from build123d import *

# Parameters (mm, degrees)
ESQUISSE1_R             = 0.9
ESQUISSE1_R_2           = 4
BOSS_EXTRU_1_DEPTH      = 6
ESQUISSE2_R             = 1.2
ENL_V_MAT_EXTRU_1_DEPTH = 10


with BuildPart() as part:
    # Esquisse1 → Boss.-Extru.1 (new body)
    with BuildSketch(Plane.XY):
        with BuildLine():
            Line((24.916434397, -77.573457495), (24.916434397, 1.426542505))
            Line((24.916434397, 1.426542505), (50.916434397, 1.426542505))
            Line((50.916434397, 1.426542505), (50.916434397, -77.573457495))
            ThreePointArc((50.916434397, -77.573457495), (49.159075085, -81.816098182), (44.916434397, -83.573457495))
            Line((44.916434397, -83.573457495), (30.916434397, -83.573457495))
            ThreePointArc((30.916434397, -83.573457495), (26.67379371, -81.816098182), (24.916434397, -77.573457495))
        make_face()
        with Locations((29.916434397, -68.573457495)):
            Circle(ESQUISSE1_R, mode=Mode.SUBTRACT)
        with Locations((37.916434397, -60.573457495)):
            Circle(ESQUISSE1_R, mode=Mode.SUBTRACT)
        with Locations((45.916434397, -68.573457495)):
            Circle(ESQUISSE1_R, mode=Mode.SUBTRACT)
        with Locations((37.916434397, -76.573457495)):
            Circle(ESQUISSE1_R, mode=Mode.SUBTRACT)
        with Locations((37.916434397, -68.573457495)):
            Circle(ESQUISSE1_R_2, mode=Mode.SUBTRACT)
    extrude(amount=BOSS_EXTRU_1_DEPTH)

    # Esquisse2 → Enlèv. mat.-Extru.1 (cut)
    with BuildSketch(Plane(origin=(0, 0, 0), x_dir=(-1, 0, 0), z_dir=(0, 0, -1))):
        with Locations((-45.336434397, -7.573457495)):
            Circle(ESQUISSE2_R)
        with Locations((-29.416434397, -7.573457495)):
            Circle(ESQUISSE2_R)
        with Locations((-45.336434397, -23.573457495)):
            Circle(ESQUISSE2_R)
        with Locations((-29.416434397, -23.573457495)):
            Circle(ESQUISSE2_R)
    extrude(amount=-ENL_V_MAT_EXTRU_1_DEPTH, mode=Mode.SUBTRACT)


solid = part.part
Here's how the part is built. I have some questions about the finished solid (model axes, mm). Give positions to 0.01 mm unless a question says otherwise; leave off trailing zeros. Loops run counter-clockwise (first coordinate to the right, second up) from the corner with the lowest first, then second, coordinate; pieces in that order, holes last. Notation, with made-up numbers: (77.5, 50) -> (81.5, 50) arc R22 ccw to (81.5, 60) -> close; hole circle Ø5 at (3.5, -13). An arc over 180 degrees is marked (long way). Answer as a JSON object with one key per item and string values. Group by question number.
Item 1: Imagine slicing it at B-B on z = 1.35. Give the number of separate pieces and of enclosed holes in the cut face, then the cut area to 3 significant figures.
Item 2: Imagine slicing it at A-A on x = 40.75. Write out the boundary of the cut face in (y, z).
Item 3: I need wall thicknesses on L1, parallel to X at y = -7.5, z = 4.25; L2, parallel to Y at x = 45.75, z = 1.7; L3, parallel to X at y = -68, z = 5.2. Which ranges of each line are inside material? Lowest first, please.
Item 4: Thinking about a two-plate mould opening in Y: for faces 1 (the flat face through (24.916, -39, 3)), 2 (the cylindrical face through (46.535, -23.521, 2.958)), 3 (the flat face through (38, 1.427, 3)), which applies, pulls with the +Y half, pulls with the -Y half, needs draft (parallel to the pull), parting line crosses it, or undercut?
Item 5: Will these pins go through, and if not, where does the flat tip stop? pin 1 (1.4 mm diameter, centred on x = 29.92, y = -68.57, fed in from -Z); pin 2 (8 mm diameter, centred on x = 46, y = -19, fed in from -Z).
Answer list:
{
 "1": {"separate pieces": "1", "enclosed holes": "9", "area": "2,120 mm2"},
 "2": {"outline": "(-83.57, 0) -> (-71.4, 0) -> (-71.4, 6) -> (-83.57, 6) -> close; (-65.75, 0) -> (1.43, 0) -> (1.43, 6) -> (-65.75, 6) -> close"},
 "3": {"L1": "x = 24.92 to 28.22, 30.61 to 44.14, 46.53 to 50.92", "L2": "y = -83.52 to -69.46, -67.69 to -24.7, -22.45 to -8.7, -6.45 to 1.43", "L3": "x = 24.92 to 29.22, 30.61 to 33.96, 41.88 to 45.22, 46.61 to 50.92"},
 "4": {"face 1": "needs draft", "face 2": "undercut", "face 3": "pulls with the +Y half"},
 "5": {"pin 1": "passes through", "pin 2": "stops at z = 0"}
}
